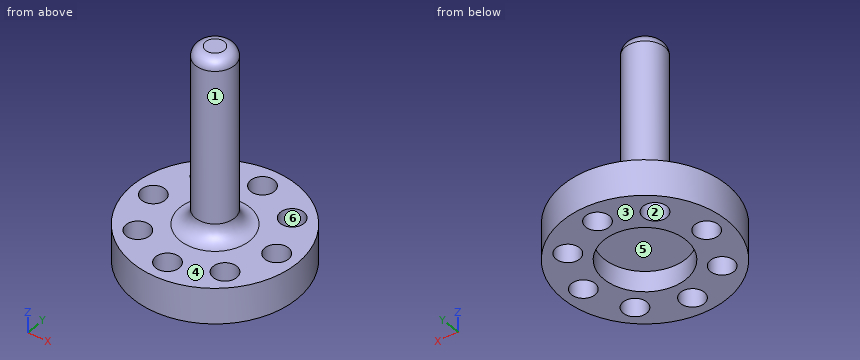
```python
from build123d import *

# Parameters (mm, degrees)
SKETCH_1_R      = 8
SKETCH_1_R_2    = 1.15
SKETCH_1_R_3    = 4
EXTRUDE_1_DEPTH = 2
SKETCH_2_R      = 8
SKETCH_2_R_2    = 1.15
EXTRUDE_2_DEPTH = 1.5
SKETCH_3_R      = 1.9
EXTRUDE_3_DEPTH = 17.5
FILLET_1_R      = 1
FILLET_2_R      = 1.5


with BuildPart() as part:
    # ｽｹｯﾁ1 → ﾎﾞｽ - 押し出し1 (new body)
    with BuildSketch(Plane.XY):
        Circle(SKETCH_1_R)
        with Locations((0, 6)):
            Circle(SKETCH_1_R_2, mode=Mode.SUBTRACT)
        with Locations((4.242640687, 4.242640687)):
            Circle(SKETCH_1_R_2, mode=Mode.SUBTRACT)
        with Locations((6, 0)):
            Circle(SKETCH_1_R_2, mode=Mode.SUBTRACT)
        with Locations((4.242640687, -4.242640687)):
            Circle(SKETCH_1_R_2, mode=Mode.SUBTRACT)
        with Locations((0, -6)):
            Circle(SKETCH_1_R_2, mode=Mode.SUBTRACT)
        with Locations((-4.242640687, -4.242640687)):
            Circle(SKETCH_1_R_2, mode=Mode.SUBTRACT)
        with Locations((-6, 0)):
            Circle(SKETCH_1_R_2, mode=Mode.SUBTRACT)
        with Locations((-4.242640687, 4.242640687)):
            Circle(SKETCH_1_R_2, mode=Mode.SUBTRACT)
        Circle(SKETCH_1_R_3, mode=Mode.SUBTRACT)
    extrude(amount=EXTRUDE_1_DEPTH)

    # ｽｹｯﾁ2 → ﾎﾞｽ - 押し出し2 (add)
    with BuildSketch(Plane.XY.offset(2)):
        Circle(SKETCH_2_R)
        with Locations((0, 6)):
            Circle(SKETCH_2_R_2, mode=Mode.SUBTRACT)
        with Locations((4.242640687, 4.242640687)):
            Circle(SKETCH_2_R_2, mode=Mode.SUBTRACT)
        with Locations((6, 0)):
            Circle(SKETCH_2_R_2, mode=Mode.SUBTRACT)
        with Locations((4.242640687, -4.242640687)):
            Circle(SKETCH_2_R_2, mode=Mode.SUBTRACT)
        with Locations((0, -6)):
            Circle(SKETCH_2_R_2, mode=Mode.SUBTRACT)
        with Locations((-4.242640687, -4.242640687)):
            Circle(SKETCH_2_R_2, mode=Mode.SUBTRACT)
        with Locations((-6, 0)):
            Circle(SKETCH_2_R_2, mode=Mode.SUBTRACT)
        with Locations((-4.242640687, 4.242640687)):
            Circle(SKETCH_2_R_2, mode=Mode.SUBTRACT)
    extrude(amount=EXTRUDE_2_DEPTH)

    # ｽｹｯﾁ3 → ﾎﾞｽ - 押し出し3 (add)
    with BuildSketch(Plane.XY.offset(3.5)):
        Circle(SKETCH_3_R)
    extrude(amount=EXTRUDE_3_DEPTH)

    # ﾌｨﾚｯﾄ1
    fillet_1_edges = [part.edges().sort_by_distance(p)[0] for p in [
        (-1.9, 0, 21),
    ]]
    fillet(fillet_1_edges, radius=FILLET_1_R)

    # ﾌｨﾚｯﾄ2
    fillet_2_edges = [part.edges().sort_by_distance(p)[0] for p in [
        (-1.9, 0, 3.5),
    ]]
    fillet(fillet_2_edges, radius=FILLET_2_R)


solid = part.part
```
Could you check a few things on this model? Use its own coordinates, in mm. Face numbers are marked on the shaded views. A direction names the side the tool comes from. Coordinates: 2 decimals unless noted, no trailing zeros. Loops run counter-clockwise (first coordinate to the right, second up) from the corner with the lowest first, then second, coordinate; pieces in that order, holes last.
1) Please list where these lines run through material, in increasing order: line 1 along X through (y, z) = (4.5, 3); line 2 along Y through (x, z) = (-6, 1.1); line 3 along Z through (x, y) = (4.5, 5.5).
Reported:
line 1: x = -6.61 to -5.36, -3.12 to 3.12, 5.36 to 6.61
line 2: y = -5.29 to -1.15, 1.15 to 5.29
line 3: z = 0 to 3.5
2) Imagine slicing it at D-D (x = 0). State how many separate pieces and enclosed holes the cut face has, and give its area (3 significant figures).
Reported:
separate pieces: 3
enclosed holes: 0
area: 90.9 mm2
3) Imagine slicing it at B-B (x = 6). List the corners of the cut face in (y, z) for me, and give its area (3 significant figures).
Reported:
outline: (-5.29, 0) - (-1.15, 0) - (-1.15, 3.5) - (-5.29, 3.5) - close; (1.15, 0) - (5.29, 0) - (5.29, 3.5) - (1.15, 3.5) - close
area: 29.0 mm2
4) Which directions (+Z, -Z, +X, -X, +Y, -Y) give clear straight access to the entire face, cutting with the end or side of a thin tool? Please do the marked faces 4, 5 and 6.
Reported:
face 4: +Z
face 5: -Z
face 6: +Z, -Z
5) Will these pins go through, and if not, where does the flat tip stop? pin 1 Ø1.5 at (x, y) = (-6.5, 5) entering from +Z; pin 2 Ø3 at (y, z) = (-3, 3.5) entering from -X; pin 3 Ø8 at (y, z) = (-5.5, 6.5) entering from +X.
Reported:
pin 1: stops at z = 3.5
pin 2: stops at x = -7.86
pin 3: stops at x = 7.47
6) Imagine slicing it at A-A (y = 4.5). List the corners of the cut face in (x, z) for me, and give its area (3 significant figures).
Reported:
outline: (-6.61, 0) - (-5.36, 0) - (-5.36, 3.5) - (-6.61, 3.5) - close; (-3.12, 0) - (3.12, 0) - (3.12, 3.5) - (-3.12, 3.5) - close; (5.36, 0) - (6.61, 0) - (6.61, 3.5) - (5.36, 3.5) - close
area: 30.6 mm2
7) Thinking about a two-plate mould opening in Y: for the marked faces 1, 2 and 3, which applies, released by +Y, released by -Y, zero draft, split by the parting line, or undercut?
Reported:
face 1: split by the parting line
face 2: undercut
face 3: zero draft
